Input: dimensioned drawing with shaded views. Units: mm. Origin: part minimum x, y, z. A direction names the side the tool comes from. Round coordinates to 2 decimals unless told otherwise and drop trailing zeros. Loops run counter-clockwise (first coordinate to the right, second up) from the corner with the lowest first, then second, coordinate; pieces in that order, holes last. Notation, with made-up numbers: (24.25, -26) - (68.25, -26) arc R32 cw to (68.25, 4) - close; hole circle Ø10 at (71, 0). An arc over 180 degrees is marked (long way). One line per question, with ' | ' between items. Start each with the question number.
1. Cut plane B-B (x = 20). Return loops of the section in (y, z).
2. Cut plane C-C (x = 5). Return loops of the section in (y, z) (1 decimal).
3. Cut plane D-D (z = 26). Return loops of the section in (x, y).
4. Ray query, line 1 (Y direction, x = 10, z = 32.5); line 2 (Y direction, x = 20, z = 32.2); line 3 (X direction, y = 16.5, z = 25.5). Return the intervals inside material, ascending.
5. Mould query, pull axis Z, two halves, no side actions, for the marked faces 3, 4, 5 and 6. Classes: pulls with the +Z half, pulls with the -Z half, needs draft (parallel to the pull), parting line crosses it, or undercut.
6. Access query for the marked faces 1 and 2. Directions: +Z, -Z, +X, -X, +Y, -Y. A direction counts if a zero-diameter tool reaches every point of the face in a straight line with its end or side. Return the directions, or none.
7. Pin query (flat end, axial travel): pin 1 (3 mm diameter, centred on y = 19.5, z = 15.5, fed in from +X); pin 2 (4 mm diameter, centred on y = 22, z = 11, fed in from +X); pin 3 (10 mm diameter, centred on x = 22, y = 12, fed in from -Z); pin 4 (3 mm diameter, centred on x = 20, y = 15, fed in from -Z). Return the tip coordinate at first contact, or that it passes through.
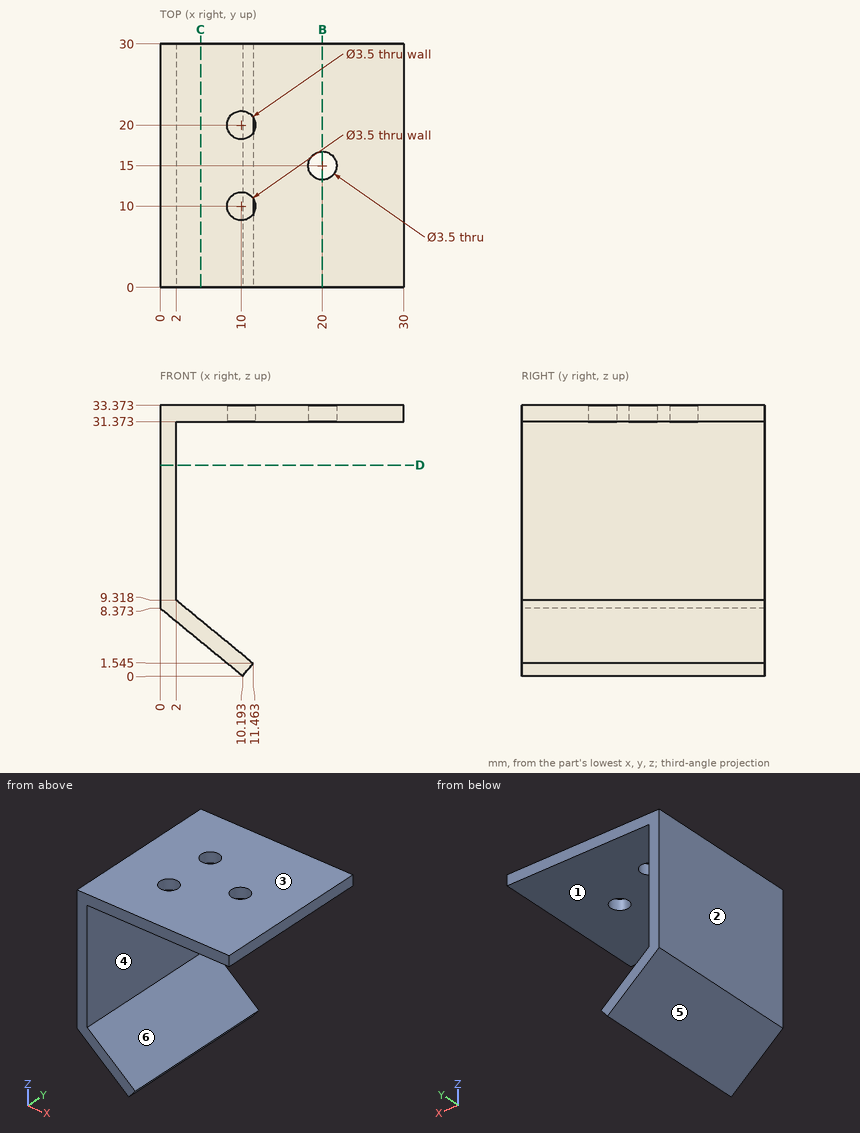
Answers follow:
1) outline: (0, 31.37) - (13.25, 31.37) - (13.25, 33.37) - (0, 33.37) - close; (16.75, 31.37) - (30, 31.37) - (30, 33.37) - (16.75, 33.37) - close
2) outline: (0, 4.3) - (30, 4.3) - (30, 6.9) - (0, 6.9) - close; (0, 31.4) - (30, 31.4) - (30, 33.4) - (0, 33.4) - close
3) outline: (0, 0) - (2, 0) - (2, 30) - (0, 30) - close
4) line 1: y = 0 to 8.25, 11.75 to 18.25, 21.75 to 30 | line 2: y = 0 to 13.25, 16.75 to 30 | line 3: x = 0 to 2
5) face 3: pulls with the +Z half | face 4: undercut | face 5: pulls with the -Z half | face 6: undercut
6) face 1: +X, +Y, -Y | face 2: +Z, -Z, -X, +Y, -Y
7) pin 1: stops at x = 2 | pin 2: stops at x = 2.39 | pin 3: stops at z = 31.37 | pin 4: passes through
